```python
from build123d import *

# Parameters (mm, degrees)
F0_R          = 17.5
F1_DEPTH      = 6.35
F3_DEPTH      = 25.4
F3_DEPTH_BACK = 25.4
F4_W          = 82.024196
F4_H          = 35
F5_DEPTH      = 6.35
F6_R          = 5.08


with BuildPart() as f1:
    # F0 (on Top) → F1 (new body)
    with BuildSketch(Plane.XY):
        Circle(F0_R)
    extrude(amount=F1_DEPTH)

    # F2 (on Front) → F3 (cut, two sides)
    with BuildSketch(Plane.XZ) as f3_sk:
        Polygon((-17.5, 0), (0, 0), (17.5, 0), (17.5, 6.171444), align=None)
    extrude(amount=F3_DEPTH, mode=Mode.SUBTRACT)
    extrude(f3_sk.sketch, amount=-F3_DEPTH_BACK, mode=Mode.SUBTRACT)

    # F4 (on face) → F5 (join)
    with BuildSketch(Plane.XY.offset(6.35)):
        with Locations((23.512098, 0)):
            Rectangle(F4_W, F4_H)
    extrude(amount=F5_DEPTH)

    # F6
    f6_edges = [f1.edges().sort_by_distance(p)[0] for p in [
        (23.512098, 17.5, 12.7),
        (-17.5, 0, 12.7),
        (23.512098, -17.5, 12.7),
        (64.524196, 0, 12.7),
    ]]
    fillet(f6_edges, radius=F6_R)


solid = f1.part
```
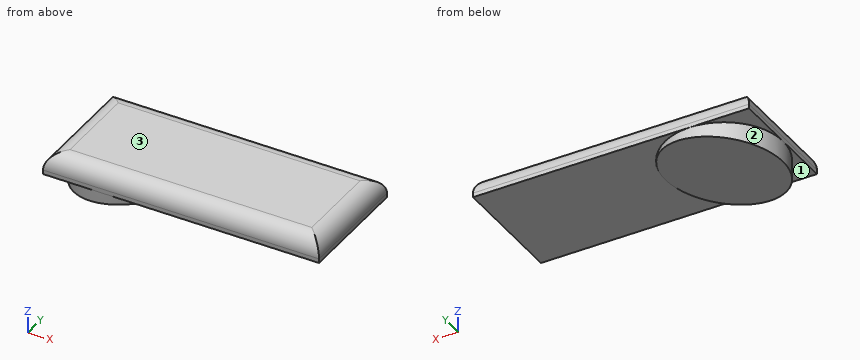
Read the model definition and answer for the solid it produces. Units are mm, in the model's axes. Face numbers are marked on the shaded views. A direction names the side the tool comes from. Round coordinates to 2 decimals unless told otherwise and drop trailing zeros. Write each loop counter-clockwise with the first axis right and the second up, starting at its lowest first coordinate (ties: lowest second). Pieces come first, ordered by that corner, then holes. Notation, with made-up numbers: (-35, 5.5) - (18, 5.5) arc R35 cw to (18, 41.5) - close; hole circle Ø11 at (-1.75, 78). An arc over 180 degrees is marked (long way). Use CSV: the item, a comma, the result in double quotes.
Q1. Find section B-B, the plane y = -8. Write down the section's boundary in (x, z).
Values:
outline,"(-17.5, 6.35) - (-15.56, 6.35) - (-15.56, 0.34) - (15.56, 5.83) - (15.56, 6.35) - (64.52, 6.35) - (64.52, 7.62) arc R5.08 ccw to (59.44, 12.7) - (-12.42, 12.7) arc R5.08 ccw to (-17.5, 7.62) - close"
Q2. Each of these flat-tipped pins is pushed along its axis until it touches: pin 1 Ø3 at (x, y) = (4, -5.5) entering from -Z; pin 2 Ø8.5 at (x, y) = (-5.5, -12) entering from -Z; pin 3 Ø10.5 at (x, y) = (26.5, -4) entering from -Z; pin 4 Ø2 at (x, z) = (40, 6) entering from +Y. Where does it stop, or does it pass through?
Values:
pin 1,"stops at z = 3.53"
pin 2,"stops at z = 1.37"
pin 3,"stops at z = 6.35"
pin 4,"stops at y = 17.5"
Q3. Straight lines are drawn through the part: line 1 along Z through (x, y) = (53, -7); line 2 along Y through (x, z) = (58.5, 7.75); line 3 along X through (y, z) = (-12.5, 7.75). For each, find the intervals that lie inside material, in ascending order.
Values:
line 1,"z = 6.35 to 12.7"
line 2,"y = -17.5 to 17.5"
line 3,"x = -17.5 to 64.52"
Q4. Find section D-D, the plane z = 10. Write down the section's boundary in (x, y), then the cut area to 3 significant figures.
Values:
outline,"(-16.91, -16.91) - (63.93, -16.91) - (63.93, 16.91) - (-16.91, 16.91) - close"
area,"2,730 mm²"
Q5. Find section C-C, the plane z = 2.5. Write down the section's boundary in (x, y), then the cut area to 3 significant figures.
Values:
outline,"(-3.32, -17.18) - (-3.32, 17.18) arc R17.5 ccw to start"
area,"365 mm²"
Q6. Find section A-A, the plane x = 8. Write down the section's boundary in (y, z), then the cut area to 3 significant figures.
Values:
outline,"(-17.5, 6.35) - (-15.56, 6.35) - (-15.56, 4.5) - (15.56, 4.5) - (15.56, 6.35) - (17.5, 6.35) - (17.5, 7.62) arc R5.08 ccw to (12.42, 12.7) - (-12.42, 12.7) arc R5.08 ccw to (-17.5, 7.62) - close"
area,"269 mm²"
Q7. A tool of negligible diameter and unlimited length cuts with its end or side. For the marked faces 1, 2 and 3, from which of +Z, -Z, +X, -X, +Y, -Y can it reach the whole face along a straight path? Write none if from no direction.
Values:
face 1,"-Z, -X, -Y"
face 2,"-Z"
face 3,"+Z, +X, -X, +Y, -Y"
